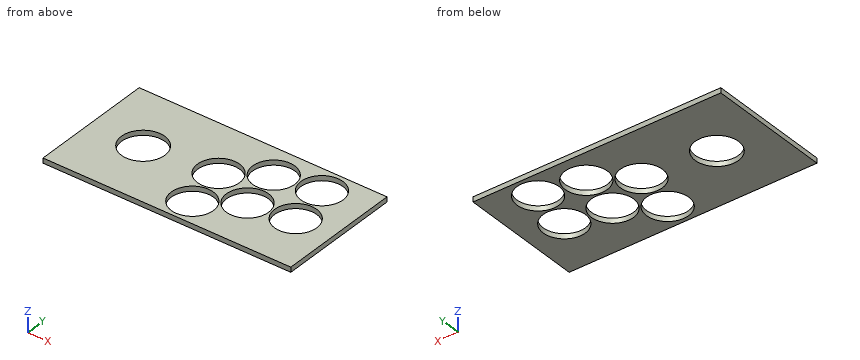
```python
from build123d import *

# Parameters (mm, degrees)
F0_W     = 200
F0_H     = 100
F2_DEPTH = 4
F1_R     = 17.5
F1_R_2   = 17
F3_DEPTH = 4


with BuildPart() as f2:
    # F0 (on Top) → F2 (new body)
    with BuildSketch(Plane.XY):
        with Locations((-32.165436, 12.314129)):
            Rectangle(F0_W, F0_H)
    extrude(amount=F2_DEPTH)

    # F1 (on face) → F3 (cut)
    with BuildSketch(Plane.XY):
        with Locations((-90.165436, 12.314129)):
            Circle(F1_R)
        with Locations((-27.165436, -17.685871)):
            Circle(F1_R_2)
        with Locations((-33.165436, 17.314129)):
            Circle(F1_R_2)
        with Locations((1.834564, 2.314129)):
            Circle(F1_R_2)
        with Locations((-4.165436, 37.314129)):
            Circle(F1_R_2)
        with Locations((36.834564, 7.314129)):
            Circle(F1_R_2)
        with Locations((30.834564, 42.314129)):
            Circle(F1_R_2)
    extrude(amount=F3_DEPTH, mode=Mode.SUBTRACT)


solid = f2.part
```
Build history of the part. All positions in model axes, mm. Round coordinates to 2 decimals unless told otherwise and drop trailing zeros. Write each loop counter-clockwise with the first axis right and the second up, starting at its lowest first coordinate (ties: lowest second). Pieces come first, ordered by that corner, then holes.
1) Pin check, flat tip, straight feed: pin 1 (6 mm diameter, centred on x = -17, y = 32.5, fed in from +Z). Stop position of the tip, or through.
2) Drill centre lines: probe 1 along Y at (x, z) = (-16, 1.85); probe 2 along X at (y, z) = (-8, 0.55); probe 3 along X at (y, z) = (51, 1.35). Where is each one in solid material? Low to high.
3) Band-saw the part on D-D, the plane y = 52. List the corners of the cut face in (x, z).
4) Band-saw the part on C-C, the plane z = 0.75. List the corners of the cut face in (x, y), and give its area (3 significant figures).
5) Band-saw the part on B-B, the plane y = -31.5. List the corners of the cut face in (x, z).
6) Band-saw the part on A-A, the plane x = 44.5. List the corners of the cut face in (y, z).
Ans:
1. pin 1: passes through
2. probe 1: y = -37.69 to -30.51, -4.87 to 25.11, 49.52 to 62.31
2. probe 2: x = -132.17 to -41.14, -13.19 to -11.68, 15.35 to 29.45, 44.22 to 67.83
2. probe 3: x = -132.17 to -14.25, 5.92 to 16.22, 45.45 to 67.83
3. outline: (-132.17, 0) - (-12.73, 0) - (-12.73, 4) - (-132.17, 4) - close; (4.4, 0) - (16.86, 0) - (16.86, 4) - (4.4, 4) - close; (44.81, 0) - (67.83, 0) - (67.83, 4) - (44.81, 4) - close
4. outline: (-132.17, -37.69) - (67.83, -37.69) - (67.83, 62.31) - (-132.17, 62.31) - close; hole circle Ø35 at (-90.17, 12.31); hole circle Ø34 at (-33.17, 17.31); hole circle Ø34 at (-27.17, -17.69); hole circle Ø34 at (-4.17, 37.31); hole circle Ø34 at (1.83, 2.31); hole circle Ø34 at (30.83, 42.31); hole circle Ø34 at (36.83, 7.31)
4. area: 13,600 mm2
5. outline: (-132.17, 0) - (-37.07, 0) - (-37.07, 4) - (-132.17, 4) - close; (-17.26, 0) - (67.83, 0) - (67.83, 4) - (-17.26, 4) - close
6. outline: (-37.69, 0) - (-7.86, 0) - (-7.86, 4) - (-37.69, 4) - close; (22.49, 0) - (32.2, 0) - (32.2, 4) - (22.49, 4) - close; (52.43, 0) - (62.31, 0) - (62.31, 4) - (52.43, 4) - close
